Model file for the job. Use its own axes, mm. Face numbers are marked on the shaded views. Give positions to 0.01 mm unless a question says otherwise; leave off trailing zeros. Loops run counter-clockwise (first coordinate to the right, second up) from the corner with the lowest first, then second, coordinate; pieces in that order, holes last. Notation, with made-up numbers: M -13,1 L 5,1 A27 cw 5,35 Z; hole C 4.5,33.25 d11. An arc over 180 degrees is marked long. Answer in a Markdown table with one row per item.
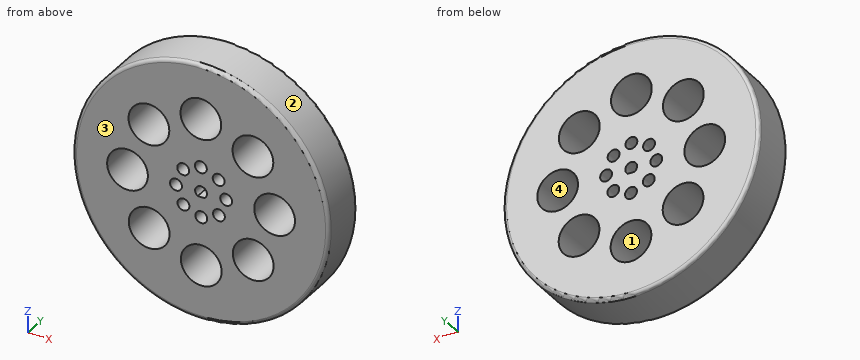
Autodesk Fusion 360 part; units mm, degrees
sketch "Sketch1" plane through (0, 0, 0) normal (0, 1, 0) x (1, 0, 0) in component "Wheel"
  circle A0 centre (0, 0) radius 55
  circle A1 centre (0.0855, 31.5759) radius 8.75
  circle A2 centre (-22.2671, 22.388) radius 8.75
  circle A3 centre (-31.5759, 0.0855) radius 8.75
  circle A4 centre (-22.388, -22.2671) radius 8.75
  circle A5 centre (-0.0855, -31.5759) radius 8.75
  circle A6 centre (22.2671, -22.388) radius 8.75
  circle A7 centre (31.5759, -0.0855) radius 8.75
  circle A8 centre (22.388, 22.2671) radius 8.75
  line L0 (-1.4465, 2.1) -> (1.4465, 2.1)
  arc A9 (-1.4465, 2.1) -> (1.4465, 2.1) centre (0, 0) ccw
  circle A10 centre (-0.0855, -10.7672) radius 2.55
  circle A11 centre (7.5531, -7.674) radius 2.55
  circle A12 centre (10.7672, -0.0855) radius 2.55
  circle A13 centre (7.674, 7.5531) radius 2.55
  circle A14 centre (0.0855, 10.7672) radius 2.55
  circle A15 centre (-7.5531, 7.674) radius 2.55
  circle A16 centre (-10.7672, 0.0855) radius 2.55
  circle A17 centre (-7.674, -7.5531) radius 2.55
  dimension "d1" = 110
  dimension "d5" = 5.1
  dimension "d6" = 17.5
  dimension "d8" = 360
  dimension "d9" = 2.1
  dimension "d12" = 5.1
  dimension "d14" = 360
extrude "Extrude2" add sketch "Sketch1" along normal blind 20 in component "Wheel"
fillet "Fillet1" radius 1.5 2 edges at (-51.278, 20, 19.8888) (-51.278, 0, 19.8888) in component "Wheel"
component "Wheel" placed x (1, 0, 0) y (0, 1, 0) z (0, 0, 1) at (0, 0, 0)
equation "d1 = ( 55 * 2 ) * 1 mm"
(1) Saw through at A-A, the plane x = 0. Give the cut face in (y, z), and give its area (3 significant figures).
Established:
| item | result |
|---|---|
| outline | M 0,-53.5 A1.5 ccw 1.5,-55 L 18.5,-55 A1.5 ccw 20,-53.5 L 20,-40.33 L 0,-40.33 Z; M 0,-22.83 L 20,-22.83 L 20,-13.32 L 0,-13.32 Z; M 0,-8.22 L 20,-8.22 L 20,-2.1 L 0,-2.1 Z; M 0,2.55 L 20,2.55 L 20,8.22 L 0,8.22 Z; M 0,13.32 L 20,13.32 L 20,22.83 L 0,22.83 Z; M 0,40.33 L 20,40.33 L 20,53.5 A1.5 ccw 18.5,55 L 1.5,55 A1.5 ccw 0,53.5 Z |
| area | 1,200 mm2 |
(2) Wall check: L1, parallel to Z at x = -26, y = 15.5; L2, parallel to X at y = 12.25, z = -17; L3, parallel to Z at x = -18, y = 12. Give the ranges that are in metal, low to high.
Established:
| item | result |
|---|---|
| L1 | z = -48.47 to -30.3, -14.47 to -6.83, 6.66 to 14.3, 30.24 to 48.47 |
| L2 | x = -52.31 to -29.16, -15.37 to 15.4, 29.38 to 52.31 |
| L3 | z = -51.97 to -30.03, -14.75 to 14.7, 29.84 to 51.97 |
(3) Flat gauge pins, fed straight in: P1, Ø4, axis at x = -7.55, z = -7.67, coming from the +Y side; P2, Ø6, axis at x = 6, y = 11.5, coming from the -Z side; P3, Ø12, axis at x = -36.5, y = 12, coming from the -Z side; P4, Ø4, axis at y = 11, z = -14, coming from the -X side. Where does each tip first touch, or does it go through?
Established:
| item | result |
|---|---|
| P1 | passes through |
| P2 | stops at z = -54.92 |
| P3 | stops at z = -45.77 |
| P4 | stops at x = -53.67 |
(4) Saw through at B-B, the plane y = 12.5. Count the separate pieces of the cut face and the enclosed holes in it, and give its area (3 significant figures).
Established:
| item | result |
|---|---|
| separate pieces | 1 |
| enclosed holes | 17 |
| area | 7,400 mm2 |
(5) Mould opens along X. For the marked faces 1, 2, 3 and 4 say: pulls with the +X half, pulls with the -X half, needs draft (parallel to the pull), parting line crosses it, or undercut.
Established:
| item | result |
|---|---|
| face 1 | undercut |
| face 2 | parting line crosses it |
| face 3 | needs draft |
| face 4 | undercut |
